The listing builds one solid part. Answer for the finished solid, in the listing's coordinates (mm). A direction names the side the tool comes from. Coordinates: 2 decimals unless noted, no trailing zeros. Write each loop counter-clockwise with the first axis right and the second up, starting at its lowest first coordinate (ties: lowest second). Pieces come first, ordered by that corner, then holes.
from build123d import *

# Parameters (mm, degrees)
SKETCH_W        = 140
SKETCH_H        = 130
SKETCH_R        = 2.35
PAD_DEPTH       = 10
SKETCH001_W     = 50
SKETCH001_H     = 50
PAD001_DEPTH    = 30
PAD002_DEPTH    = 50
FILLET_R        = 10
CHAMFER_SIZE    = 1
SKETCH003_W     = 38
SKETCH003_H     = 64.710678
POCKET_DEPTH    = 4
POCKET_TAPER    = -30
PAD003_DEPTH    = 10
SKETCH005_W     = 60
SKETCH005_H     = 9
POCKET001_DEPTH = 6
FILLET001_R     = 3


with BuildPart() as part:
    # Sketch → Pad (new body)
    with BuildSketch(Plane.XY):
        Rectangle(SKETCH_W, SKETCH_H)
        with Locations((-50, 45)):
            Circle(SKETCH_R, mode=Mode.SUBTRACT)
        with Locations((50, 45)):
            Circle(SKETCH_R, mode=Mode.SUBTRACT)
        with Locations((-50, -45)):
            Circle(SKETCH_R, mode=Mode.SUBTRACT)
        with Locations((50, -45)):
            Circle(SKETCH_R, mode=Mode.SUBTRACT)
    extrude(amount=PAD_DEPTH)

    # Sketch001 (on Face10 of Pad) → Pad001 (join)
    with BuildSketch(Plane.XY.offset(10)):
        Rectangle(SKETCH001_W, SKETCH001_H)
    extrude(amount=PAD001_DEPTH)

    # Sketch002 (on DatumPlane) → Pad002 (join)
    with BuildSketch(Plane.YZ.offset(25)):
        Polygon((-25, 40), (25, 90), (25, 40), align=None)
    extrude(amount=-PAD002_DEPTH)

    # Fillet
    fillet_edges = [part.edges().sort_by_distance(p)[0] for p in [
        (70, -65, 5),
        (70, 65, 5),
        (-70, -65, 5),
        (-70, 65, 5),
    ]]
    fillet(fillet_edges, radius=FILLET_R)

    # Chamfer
    chamfer_edges = [part.edges().sort_by_distance(p)[0] for p in [
        (-52.35, -45, 10),
        (47.65, -45, 10),
        (47.65, 45, 10),
        (-52.35, 45, 10),
    ]]
    chamfer(chamfer_edges, length=CHAMFER_SIZE)

    # Sketch003 (on Face21 of Chamfer) → Pocket (cut)
    with BuildSketch(Plane(origin=(0, -32.5, 32.5), x_dir=(1, 0, 0), z_dir=(0, -0.707107, 0.707107))):
        with Locations((0, 48.961941)):
            Rectangle(SKETCH003_W, SKETCH003_H)
    extrude(amount=-POCKET_DEPTH, taper=POCKET_TAPER, mode=Mode.SUBTRACT)

    # Sketch004 → Pad003 (join)
    with BuildSketch(Plane.YZ.offset(-65)):
        Polygon((-35, 10), (-35, 26), (25, 86), (25, 10), align=None)
    pad003 = extrude(amount=PAD003_DEPTH)

    # Mirrored: Pad003 across YZ
    add(pad003.mirror(Plane.YZ))

    # Sketch005 → Pocket001 (cut)
    with BuildSketch(Plane.XY):
        with Locations((40, 0)):
            Rectangle(SKETCH005_W, SKETCH005_H)
    extrude(amount=POCKET001_DEPTH, mode=Mode.SUBTRACT)

    # Fillet001
    fillet001_edges = [part.edges().sort_by_distance(p)[0] for p in [
        (40, 4.5, 6),
        (40, -4.5, 6),
    ]]
    fillet(fillet001_edges, radius=FILLET001_R)


solid = part.part
Q1. Determine the mould class of faces 1 (the face through (60, -35, 18)), 2 (the face through (10, 0, 3)), 3 (the face through (51.263, -43.018, 4.437)), 4 (the face through (51.263, 46.982, 4.437)) for opening direction X: released by +X, released by -X, zero draft, split by the parting line, or undercut.
Answers below:
face 1: zero draft
face 2: released by +X
face 3: undercut
face 4: undercut
Q2. Given pin 1 (8 mm diameter, centred on x = 9.5, y = -31.5, fed in from -Z); pin 2 (3 mm diameter, centred on x = 62.5, z = 31, fed in from +Y); pin 3 (25 mm diameter, centred on y = 2, z = 55.5, fed in from +X); pin 4 (1.8 mm diameter, centred on y = 2, z = 2.5, fed in from +X), each flat-ended and moving along its own axis, determine where each tip first touches the part or whether it passes through.
Answers below:
pin 1: stops at z = 0
pin 2: stops at y = 25
pin 3: stops at x = 65
pin 4: stops at x = 10
Q3. Which of the six approach directions +Z, -Z, +X, -X, +Y, -Y give full straight-line access (tool end or side, diameter ignored) to faces 5 (the face through (-60, 25, 49)), 6 (the face through (-60, -5, 56)), 7 (the face through (-60, -35, 18))?
Answers below:
face 5: +Z, +X, -X, +Y
face 6: +Z, -X, -Y
face 7: +Z, +X, -X, -Y
Q4. The part is cut by section A-A, the plane x = 50. Write down the section's boundary in (y, z), then the cut area to 3 significant figures.
Answers below:
outline: (-65, 0) - (-47.35, 0) - (-47.35, 9) - (-48.35, 10) - (-65, 10) - close; (-42.65, 0) - (-4.5, 0) - (-4.5, 3) arc R3 cw to (-1.5, 6) - (1.5, 6) arc R3 cw to (4.5, 3) - (4.5, 0) - (42.65, 0) - (42.65, 9) - (41.65, 10) - (-41.65, 10) - (-42.65, 9) - close; (47.35, 0) - (65, 0) - (65, 10) - (48.35, 10) - (47.35, 9) - close
area: 1,150 mm2
Q5. The part is cut by section C-C, the plane x = -50. Write down the section's boundary in (y, z).
Answers below:
outline: (-65, 0) - (-47.35, 0) - (-47.35, 9) - (-48.35, 10) - (-65, 10) - close; (-42.65, 0) - (42.65, 0) - (42.65, 9) - (41.65, 10) - (-41.65, 10) - (-42.65, 9) - close; (47.35, 0) - (65, 0) - (65, 10) - (48.35, 10) - (47.35, 9) - close
Q6. The part is cut by section B-B, the plane y = 45. Write down the section's boundary in (x, z).
Answers below:
outline: (-70, 0) - (-52.35, 0) - (-52.35, 9) - (-53.35, 10) - (-70, 10) - close; (-47.65, 0) - (47.65, 0) - (47.65, 9) - (46.65, 10) - (-46.65, 10) - (-47.65, 9) - close; (52.35, 0) - (70, 0) - (70, 10) - (53.35, 10) - (52.35, 9) - close
Q7. Find the intervals of material crossed by probe 1 along X at (y, z) = (12, 31.5); probe 2 along Y at (x, z) = (-50, 5); probe 3 along Y at (x, z) = (50, 2.25), in increasing order.
Answers below:
probe 1: x = -65 to -55, -25 to 25, 55 to 65
probe 2: y = -65 to -47.35, -42.65 to 42.65, 47.35 to 65
probe 3: y = -65 to -47.35, -42.65 to -4.5, 4.5 to 42.65, 47.35 to 65
